Can you work these out from the model? Positions are in its coordinate system, mm. Face numbers are marked on the shaded views. A direction names the side the tool comes from. Give positions to 0.01 mm unless a question says otherwise; leave off trailing zeros. Write each loop counter-clockwise with the first axis right and the second up, starting at its lowest first coordinate (ties: lowest second). Pieces come first, ordered by that corner, then holes. Notation, with made-up numbers: (-39, 54.25) - (0, 54.25) arc R18 ccw to (0, 63.25) - close; hole circle Ø8 at (71.25, 24.5). An arc over 180 degrees is marked (long way). Return JSON: item names as keys, results as strings. Group by question number.
from build123d import *

# Parameters (mm, degrees)
SKETCH1_R           = 2.2479
BOSS_EXTRUDE1_DEPTH = 36.3982
BOSS_EXTRUDE2_DEPTH = 2.921
SKETCH3_R           = 18.5801
BOSS_EXTRUDE3_DEPTH = 5.8674
FILLET1_R           = 2.54
SKETCH4_R           = 8.4709
BOSS_EXTRUDE4_DEPTH = 4.7244
FILLET2_R           = 2.54


with BuildPart() as part:
    # Sketch1 → Boss-Extrude1 (new body)
    with BuildSketch(Plane(origin=(0, 0, 0), x_dir=(0, 0, -1), z_dir=(1, 0, 0))):
        Circle(SKETCH1_R)
    extrude(amount=BOSS_EXTRUDE1_DEPTH)

    # Sketch2 → Boss-Extrude2 (add)
    with BuildSketch(Plane(origin=(27.5082, 0, 0), x_dir=(0, 0, -1), z_dir=(1, 0, 0))):
        with BuildLine():
            Line((0, -1.334463955), (-13.814144421, 6.641136045))
            Line((-13.814144421, 6.641136045), (-26.133144421, 6.641136045))
            ThreePointArc((-26.133144421, 6.641136045), (-12.195347715, 7.850704504), (0, 0.995142749))
            Line((0, 0.995142749), (0, -1.334463955))
        make_face()
    extrude(amount=-BOSS_EXTRUDE2_DEPTH)

    # Sketch3 → Boss-Extrude3 (add)
    with BuildSketch(Plane.XZ.offset(-6.641136045)):
        with Locations(Location((26.0477, 32.394244421, 0), (0, 0, 270))):
            Circle(SKETCH3_R)
    extrude(amount=BOSS_EXTRUDE3_DEPTH)

    # Fillet1
    fillet1_edges = [part.edges().sort_by_distance(p)[0] for p in [
        (26.0477, 6.641136045, 50.974344421),
        (26.0477, 0.773736045, 50.974344421),
    ]]
    fillet(fillet1_edges, radius=FILLET1_R)

    # Sketch4 → Boss-Extrude4 (add)
    with BuildSketch(Plane(origin=(0, 6.641136045, 0), x_dir=(1, 0, 0), z_dir=(0, 1, 0))):
        with Locations(Location((26.0477, -38.248526032, 0), (0, 0, 90))):
            Circle(SKETCH4_R)
    extrude(amount=BOSS_EXTRUDE4_DEPTH)

    # Fillet2
    fillet2_edges = [part.edges().sort_by_distance(p)[0] for p in [
        (26.0477, 11.365536045, 46.719426032),
    ]]
    fillet(fillet2_edges, radius=FILLET2_R)


solid = part.part
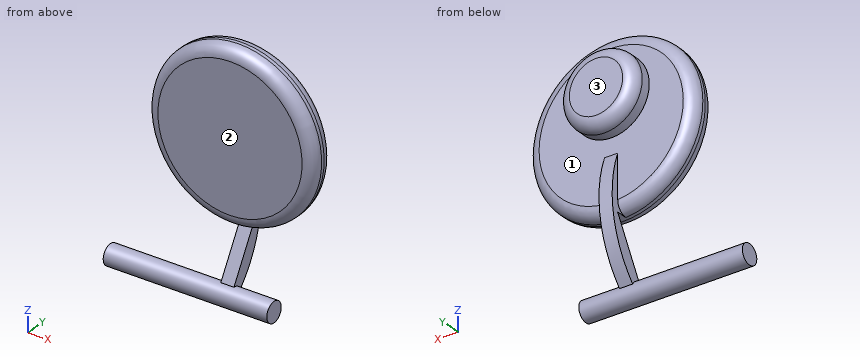
1) Imagine slicing it at D-D, the plane y = -1. Write out the boundary of the cut face in (x, z), and give its area (3 significant figures).
2) Will these pins go through, and if not, where does the flat tip stop? pin 1 Ø4 at (x, z) = (9, 22) entering from -Y; pin 2 Ø1.5 at (y, z) = (2, 10) entering from -X; pin 3 Ø5 at (y, z) = (1, 0) entering from +X; pin 4 Ø3 at (x, y) = (14.5, 4) entering from +Z.
3) I need wall thicknesses on line 1 along Y through (x, z) = (35.5, 41.5); line 2 along X through (y, z) = (4.5, 8); line 3 along Z through (x, y) = (31.5, -0.25). Which ranges of each line are inside material? Lowest first, please.
4) Imagine slicing it at B-B, the plane y = 7.5. Write out the boundary of the cut face in (x, z), and give its area (3 significant figures).
5) Imagine slicing it at C-C, the plane x = 4.5. Write out the boundary of the cut face in (y, z).
6) Imagine slicing it at A-A, the plane z = 0. Write out the boundary of the cut face in (x, y).
7) On a 3-axis mill with a long thin cutter (end or side, diameter ignored), from which of +Z, -Z, +X, -X, +Y, -Y can I reach the whole of each face in a straight line? I mean the marked faces 1, 2 and 3. Say none if no direction works.
Resolved:
{
 "1": {"outline": "(0, -2.01) - (36.4, -2.01) - (36.4, 2.01) - (0, 2.01) - close", "area": "147 mm^2"},
 "2": {"pin 1": "y = 1.66", "pin 2": "through", "pin 3": "x = 36.4", "pin 4": "z = 48.02"},
 "3": {"line 1": "0.77 to 6.64", "line 2": "24.59 to 27.51", "line 3": "-2.23 to 2.23"},
 "4": {"outline": "circle Ø16.94 at (26.05, 38.25); (24.59, 10.78) - (27.51, 10.78) - (27.51, 23.63) - (24.59, 23.63) - close", "area": "263 mm^2"},
 "5": {"outline": "circle Ø4.5 at (0, 0)"},
 "6": {"outline": "(0, -2.25) - (36.4, -2.25) - (36.4, 2.25) - (0, 2.25) - close"},
 "7": {"face 1": "+Y", "face 2": "+Z, +X, -X, -Y", "face 3": "+Z, -Z, +X, -X, +Y"}
}
